Can you work these out from the drawing? Everything is in mm from the part's minimum corner. A direction names the side the tool comes from. Coordinates: 2 decimals unless noted, no trailing zeros. Order: outer loops, then holes, each group sorted by start corner. A loop starts at its lowest first (then second) coordinate and runs counter-clockwise, first axis right, second up. Notation, with made-up numbers: (26.25, 37) -> (46.25, 37) arc R17 ccw to (46.25, 66) -> close; hole circle Ø5 at (39.5, 12). An arc over 180 degrees is marked (long way). Put each result on its own line as item: value. Start each with the question number.
Q1. For the marked faces 1, 2, 3, 4 and 5, which set-ups out of +Z, -Z, +X, -X, +Y, -Y let a thin tool reach every point of the face, with its end or its side?
Q2. If we section it at C-C (z = 36): Please give me the cut outline in (x, y) (1 decimal).
Q3. If we section it at A-A (y = 22.5): Please give me the cut outline in (x, z).
Q4. Will these pins go through, and if not, where does the flat tip stop? pin 1 (2 mm diameter, centred on x = 22.5, z = 31, fed in from +Y) (1 decimal); pin 2 (20 mm diameter, centred on y = 25.5, z = 39, fed in from -X); pin 3 (6 mm diameter, centred on x = 44, z = 40, fed in from +Y).
Q5. Please list where these lines run through material, in increasing order: line 1 along Z through (x, y) = (9.5, 42.5); line 2 along X through (y, z) = (9, 42.5); line 3 along Y through (x, z) = (25, 36) (1 decimal).
Q6. If we section it at B-B (x = 34): Please give me the cut outline in (y, z) (1 decimal).
Q7. If we section it at D-D (x = 8): Please give me the cut outline in (y, z), and give its area (3 significant figures).
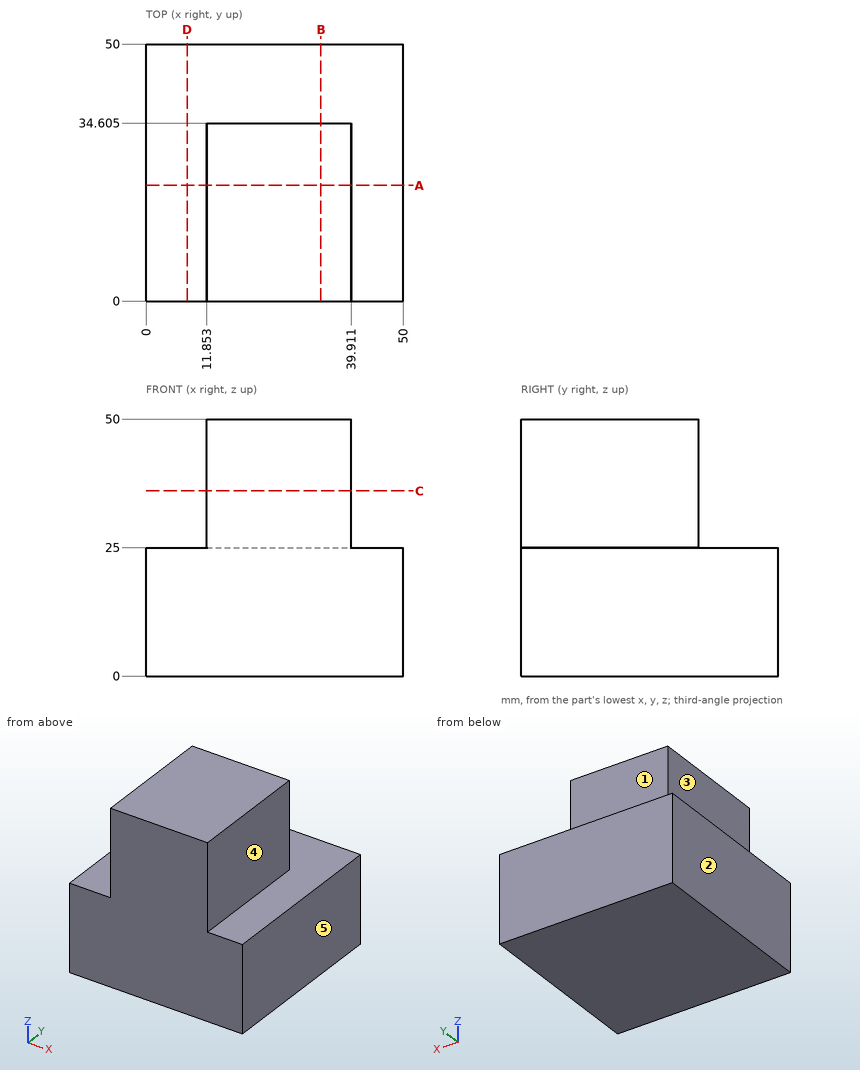
The answers:
1. face 1: +Z, +X, -X, +Y
1. face 2: +Z, -Z, -X, +Y, -Y
1. face 3: +Z, -X, +Y, -Y
1. face 4: +Z, +X, +Y, -Y
1. face 5: +Z, -Z, +X, +Y, -Y
2. outline: (11.9, 0) -> (39.9, 0) -> (39.9, 34.6) -> (11.9, 34.6) -> close
3. outline: (0, 0) -> (50, 0) -> (50, 25) -> (39.91, 25) -> (39.91, 50) -> (11.85, 50) -> (11.85, 25) -> (0, 25) -> close
4. pin 1: y = 34.6
4. pin 2: x = 11.85
4. pin 3: through
5. line 1: 0 to 25
5. line 2: 11.85 to 39.91
5. line 3: 0 to 34.6
6. outline: (0, 0) -> (50, 0) -> (50, 25) -> (34.6, 25) -> (34.6, 50) -> (0, 50) -> close
7. outline: (0, 0) -> (50, 0) -> (50, 25) -> (0, 25) -> close
7. area: 1,250 mm^2
